Geometry check sheet. Reference: the model listing, model coordinates, mm. Face numbers are marked on the shaded views. Give positions to 0.01 mm unless a question says otherwise; leave off trailing zeros. Order: outer loops, then holes, each group sorted by start corner. A loop starts at its lowest first (then second) coordinate and runs counter-clockwise, first axis right, second up. Notation, with made-up numbers: M 60.5,76.25 L 107.5,76.25 A11 cw 107.5,94.25 Z; hole C 79.5,69.5 d6. An arc over 180 degrees is marked long. Answer as CSV lines item,"result".
from build123d import *

# Parameters (mm, degrees)
SKETCH_R     = 10
PAD_DEPTH    = 3
SKETCH001_R  = 6.5
PAD001_DEPTH = 15
SKETCH002_R  = 3.5
POCKET_DEPTH = 15
FILLET_R     = 2
CHAMFER_SIZE = 2


with BuildPart() as part:
    # Sketch → Pad (new body)
    with BuildSketch(Plane.XY):
        Circle(SKETCH_R)
    extrude(amount=PAD_DEPTH)

    # Sketch001 (on Face3 of Pad) → Pad001 (join)
    with BuildSketch(Plane.XY.offset(3)):
        Circle(SKETCH001_R)
    extrude(amount=PAD001_DEPTH)

    # Sketch002 (on Face5 of Pad001) → Pocket (cut)
    with BuildSketch(Plane.XY.offset(18)):
        Circle(SKETCH002_R)
    extrude(amount=-POCKET_DEPTH, mode=Mode.SUBTRACT)

    # Fillet
    fillet_edges = [part.edges().sort_by_distance(p)[0] for p in [
        (-10, 0, 0),
    ]]
    fillet(fillet_edges, radius=FILLET_R)

    # Chamfer
    chamfer_edges = [part.edges().sort_by_distance(p)[0] for p in [
        (-6.5, 0, 18),
    ]]
    chamfer(chamfer_edges, length=CHAMFER_SIZE)


solid = part.part
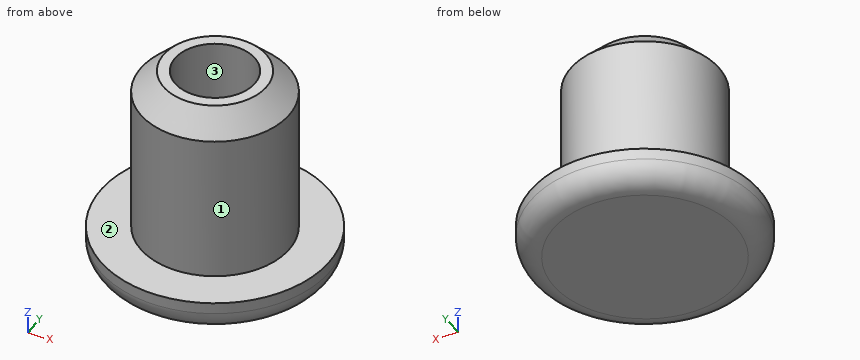
(1) Section check C-C on z = 13.5. Enter the section's corners in (x, y).
The answers:
outline,"C 0,0 d13; hole C 0,0 d7"
(2) Draft check along X on the marked faces 1, 2 and 3. Enter one of: +X half, -X half, draft (parallel to the pull), parting line (faces both ways), or undercut.
The answers:
face 1,"parting line"
face 2,"draft"
face 3,"undercut"
(3) Section check A-A on x = 0. Enter the section's corners in (y, z), then the cut area to 3 significant figures.
The answers:
outline,"M -10,2 A2 ccw -8,0 L 8,0 A2 ccw 10,2 L 10,3 L 6.5,3 L 6.5,16 L 4.5,18 L 3.5,18 L 3.5,3 L -3.5,3 L -3.5,18 L -4.5,18 L -6.5,16 L -6.5,3 L -10,3 Z"
area,"144 mm2"
(4) Gauge pin test, flat ends, axial feed: P1, Ø6, axis at x = 1, y = 6, coming from the +Z side; P2, Ø6, axis at x = -6.5, z = 3, coming from the -Y side; P3, Ø1.5, axis at x = 1, z = 3, coming from the -Y side; P4, Ø1.5, axis at x = -6.5, y = 3.5, coming from the +Z side. Record the tip position at first contact, or that the pin passes through.
The answers:
P1,"stops at z = 18"
P2,"stops at y = -9.37"
P3,"stops at y = -10"
P4,"stops at z = 3"
(5) Material ranges on line 1 (Y direction, x = 0, z = 6); line 2 (X direction, y = 0.75, z = 16.25); line 3 (X direction, y = -1.5, z = 9), recorded low to high.
The answers:
line 1,"y = -6.5 to -3.5, 3.5 to 6.5"
line 2,"x = -6.2 to -3.42, 3.42 to 6.2"
line 3,"x = -6.32 to -3.16, 3.16 to 6.32"
(6) Section check D-D on z = 1.5. Enter the section's corners in (x, y).
The answers:
outline,"C 0,0 d19.87"
